```python
from build123d import *

# Parameters (mm, degrees)
F0_W      = 47.5
F0_H      = 35
F1_DEPTH  = 17
F2_W      = 37.5
F2_H      = 35
F3_DEPTH  = 10
F5_DEPTH  = 10.001
F6_W      = 22.5
F6_H      = 2.5
F7_DEPTH  = 7.001
F9_DEPTH  = 7.001
F11_DEPTH = 7.001


with BuildPart() as f1:
    # F0 (on Top) → F1 (new body)
    with BuildSketch(Plane.XY):
        with Locations((-79.0966801345, -8.9940691388)):
            Rectangle(F0_W, F0_H)
    extrude(amount=F1_DEPTH)

    # F2 (on face) → F3 (cut)
    with BuildSketch(Plane.XY.offset(17)):
        with Locations((-74.0966801345, -8.9940691388)):
            Rectangle(F2_W, F2_H)
    extrude(amount=-F3_DEPTH, mode=Mode.SUBTRACT)

    # F4 (on face) → F5 (cut, through all)
    with BuildSketch(Plane.YZ.offset(-92.8466801345)):
        Polygon((1.0059308612, 17), (-18.9940691388, 17), (-21.4939605839, 13.7453228235), (3.5060394161, 13.7453228235), align=None)
    extrude(amount=-F5_DEPTH, mode=Mode.SUBTRACT)

    # F6 (on face) → F7 (cut, through all)
    with BuildSketch(Plane.XY.offset(7)):
        with Locations((-66.5966801345, -7.7440691388)):
            Rectangle(F6_W, F6_H)
    extrude(amount=-F7_DEPTH, mode=Mode.SUBTRACT)

    # F8 (on face) → F9 (cut, through all)
    with BuildSketch(Plane.XY.offset(7)):
        Polygon((-55.3466801345, 8.5059308612), (-67.8466801345, 8.5059308612), (-55.3466801345, -2.4940691388), align=None)
    extrude(amount=-F9_DEPTH, mode=Mode.SUBTRACT)

    # F10 (on face) → F11 (cut, through all)
    with BuildSketch(Plane.XY.offset(7)):
        Polygon((-55.3466801345, -26.4940691388), (-55.3466801345, -12.9940691388), (-67.8466801345, -26.4940691388), align=None)
    extrude(amount=-F11_DEPTH, mode=Mode.SUBTRACT)


solid = f1.part
```
Geometry: final body of the model. Coordinates: model frame, mm. A direction names the side the tool comes from. Coordinates: 2 decimals unless noted, no trailing zeros. Order: outer loops, then holes, each group sorted by start corner. A loop starts at its lowest first (then second) coordinate and runs counter-clockwise, first axis right, second up.
Item 1: Section query D-D (y = -9.5). Output: boundary loops of the cut face in (x, z).
Answer:
outline: (-102.85, 0) - (-55.35, 0) - (-55.35, 7) - (-92.85, 7) - (-92.85, 13.75) - (-102.85, 13.75) - close
Item 2: Material intervals for line 1 along Y through (x, z) = (-68, 6.5); line 2 along Z through (x, y) = (-96.5, -20); line 3 along X through (y, z) = (-24, 10.75), sorted ascending.
Answer:
line 1: y = -26.49 to -8.99, -6.49 to 8.51
line 2: z = 0 to 13.75, 15.69 to 17
line 3: x = -102.85 to -92.85
Item 3: Draft query along Y for faces 1 (the face through (-89, -26.494, 6)), 2 (the face through (-67, -8.994, 4)), 3 (the face through (-61.68, 3.08, 3.55)). Return one class per face: released by +Y, released by -Y, zero draft, split by the parting line, or undercut.
Answer:
face 1: released by -Y
face 2: undercut
face 3: released by +Y
Item 4: Section query A-A (x = -73). Output: boundary loops of the cut face in (y, z).
Answer:
outline: (-26.49, 0) - (-8.99, 0) - (-8.99, 7) - (-26.49, 7) - close; (-6.49, 0) - (8.51, 0) - (8.51, 7) - (-6.49, 7) - close
Item 5: Contact query for flat-ended pins moving along their axis: P1, Ø2, axis at x = -73, y = -15.5, coming from the +Z side; P2, Ø8, axis at x = -99.5, y = -8.5, coming from the +Z side; P3, Ø5.5, axis at x = -61.5, z = 2.5, coming from the +Y side. Output: stop coordinate, or through.
Answer:
P1: stops at z = 7
P2: stops at z = 13.75
P3: stops at y = 5.34
Item 6: Section query C-C (z = 15.5). Output: boundary loops of the cut face in (x, y).
Answer:
outline: (-102.85, -26.49) - (-92.85, -26.49) - (-92.85, -20.15) - (-102.85, -20.15) - close; (-102.85, 2.16) - (-92.85, 2.16) - (-92.85, 8.51) - (-102.85, 8.51) - close
Item 7: Access query for faces 4 (the face through (-92.847, -9, 11)), 5 (the face through (-89, 8.506, 6)), 6 (the face through (-98, -9, 13.745)), 7 (the face through (-55.347, -5, 3)), 8 (the face through (-67, -6.494, 4)). Directions: +Z, -Z, +X, -X, +Y, -Y. A direction counts if a zero-diameter tool reaches every point of the face in a straight line with its end or side. Return the directions, or none.
Answer:
face 4: +Z, +X, +Y, -Y
face 5: +Z, -Z, +X, -X, +Y
face 6: +X, -X
face 7: +Z, -Z, +X, +Y, -Y
face 8: +Z, -Z, +X
Item 8: Section query B-B (z = 1.75). Output: boundary loops of the cut face in (x, y).
Answer:
outline: (-102.85, -26.49) - (-67.85, -26.49) - (-55.35, -12.99) - (-55.35, -8.99) - (-77.85, -8.99) - (-77.85, -6.49) - (-55.35, -6.49) - (-55.35, -2.49) - (-67.85, 8.51) - (-102.85, 8.51) - close
